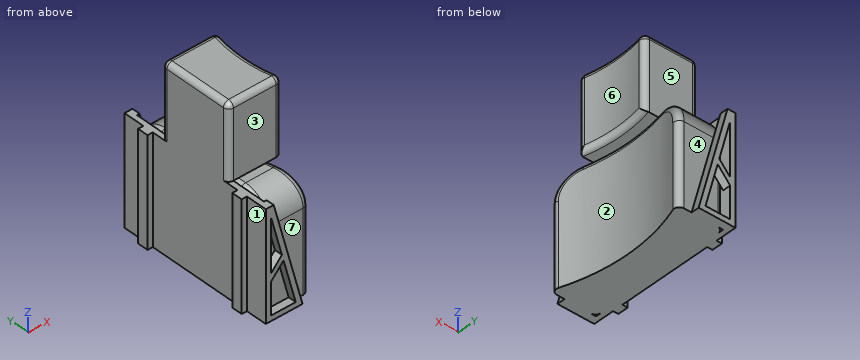
```python
from build123d import *

# Parameters (mm, degrees)
F1_DEPTH  = 15
F2_W      = 7
F2_H      = 27
F3_DEPTH  = 25
F6_DEPTH  = 20
F8_W      = 1
F8_H      = 2
F9_DEPTH  = 20.5262794416
F10_W     = 9
F10_H     = 27
F11_DEPTH = 20.5262794416
F12_R     = 35.75
F13_DEPTH = 30
F15_R     = 5
F16_R     = 1
F17_W     = 11
F17_H     = 14
F18_DEPTH = 14
F19_R     = 27.5
F20_DEPTH = 60
F22_R     = 1


with BuildPart() as f1:
    # F0 (on Front) → F1 (new body, symmetric)
    with BuildSketch(Plane.XZ):
        Polygon((0, 20.5262794416), (0, 0), (7, 0), (1.5, 20.5262794416), align=None)
    extrude(amount=F1_DEPTH, both=True)


with BuildPart() as f3:
    # F2 (on Top) → F3 (new body)
    with BuildSketch(Plane.XY):
        with Locations((4.5, 0)):
            Rectangle(F2_W, F2_H)
    extrude(amount=F3_DEPTH)


with BuildPart() as f6:
    # F4 (on Front) → F6 (new body, symmetric)
    with BuildSketch(Plane.XZ):
        Polygon((3.0705523608, 10.8011949299), (1, 18.5286015403), (1, 8.5286015403), align=None)
    extrude(amount=F6_DEPTH, both=True)


with BuildPart() as f6b:
    # F5 (on Front) → F6, piece 2 (new body, symmetric)
    with BuildSketch(Plane.XZ):
        Polygon((3.377991262, 9.6538173306), (1, 7.0437856671), (1, 1), (5.6967746272, 1), align=None)
    extrude(amount=F6_DEPTH, both=True)


with BuildPart() as f1_1:
    add(f1.part)

    # F7: cut F6b, F6, F3
    add(f6b.part, mode=Mode.SUBTRACT)
    add(f6.part, mode=Mode.SUBTRACT)
    add(f3.part, mode=Mode.SUBTRACT)

    # F8 (on face) → F9 (join, through all)
    with BuildSketch(Plane.XY.offset(20.5262794416)):
        with Locations((-0.5, -10)):
            Rectangle(F8_W, F8_H)
        with Locations((-0.5, 10)):
            Rectangle(F8_W, F8_H)
    extrude(amount=-F9_DEPTH)



with BuildPart() as f11:
    # F10 (on Top) → F11 (new body, through all)
    with BuildSketch(Plane.XY):
        with Locations((5.5, 0)):
            Rectangle(F10_W, F10_H)
    extrude(amount=F11_DEPTH)


with BuildPart() as f13:
    # F12 (on Top) → F13 (new body)
    with BuildSketch(Plane.XY):
        with Locations((43, 0)):
            Circle(F12_R)
    extrude(amount=F13_DEPTH)


with BuildPart() as f11_1:
    add(f11.part)

    # F14: cut F13
    add(f13.part, mode=Mode.SUBTRACT)

    # F15
    f15_edges = [f11_1.edges().sort_by_distance(p)[0] for p in [
        (5.448471, -13.5, 20.526279),
        (5.448471, 13.5, 20.526279),
    ]]
    fillet(f15_edges, radius=F15_R)

    # F16
    f16_edges = [f11_1.edges().sort_by_distance(p)[0] for p in [
        (9.896941, -13.5, 7.76314),
        (1, -13.5, 7.76314),
    ]]
    fillet(f16_edges, radius=F16_R)


with BuildPart() as f1_2:
    add(f1_1.part)

    add(f11_1.part)  # F18 merges F11
    # F17 (on face) → F18 (join)
    with BuildSketch(Plane.XY.offset(20.5262794416)):
        with Locations((5.5, 0)):
            Rectangle(F17_W, F17_H)
    extrude(amount=F18_DEPTH)


with BuildPart() as f20:
    # F19 (on Top) → F20 (new body)
    with BuildSketch(Plane.XY):
        with Locations((37, 0)):
            Circle(F19_R)
    extrude(amount=F20_DEPTH)


with BuildPart() as f1_3:
    add(f1_2.part)

    # F21: cut F20
    add(f20.part, mode=Mode.SUBTRACT)

    # F22
    f22_edges = [f1_3.edges().sort_by_distance(p)[0] for p in [
        (10.405828, 7, 27.526279),
        (9.5, 0, 20.526279),
        (10.405828, -7, 27.526279),
        (9.5, 0, 34.526279),
        (5.202914, 7, 34.526279),
        (5.202914, -7, 34.526279),
        (0, 0, 34.526279),
        (0, 7, 27.526279),
        (0, -7, 27.526279),
    ]]
    fillet(f22_edges, radius=F22_R)


solid = f1_3.part
```
Model file for the job. Use its own axes, mm. Face numbers are marked on the shaded views. A direction names the side the tool comes from. Give positions to 0.01 mm unless a question says otherwise; leave off trailing zeros. Loops run counter-clockwise (first coordinate to the right, second up) from the corner with the lowest first, then second, coordinate; pieces in that order, holes last. Notation, with made-up numbers: M 65,75.5 L 77,75.5 A21 ccw 77,110.5 Z; hole C 2.25,19.5 d9. An arc over 180 degrees is marked long. Use one line per item in the form item = value.
Item 1: Which spindle directions (+Z, -Z, +X, -X, +Y, -Y) get a long thin tool onto all of the face, cutting with end or side? Do the marked faces 1, 2, 3 and 4. Say none if no direction does.
Filled in:
face_1 = +Z, -Z, -X, -Y
face_2 = -Z, +X
face_3 = +Z, +X, -X, -Y
face_4 = +Z, +X, +Y
Item 2: Flat gauge pins, fed straight in: pin 1 Ø1.2 at (x, y) = (5.5, -8) entering from +Z; pin 2 Ø1.5 at (x, z) = (4.5, 23) entering from -Y; pin 3 Ø4 at (y, z) = (2.5, 25) entering from +X. Where does each tip first touch, or does it go through?
Filled in:
pin_1 = 20.53
pin_2 = -7
pin_3 = 9.87
Item 3: Drill centre lines: L1, parallel to Y at x = -0.25, z = 10.5; L2, parallel to X at y = 8.5, z = 12.5; L3, parallel to X at y = -9.5, z = 10. Where is each one in solid material? Low to high.
Filled in:
L1 = -11 to -9, 9 to 11
L2 = 0 to 8.28
L3 = -1 to 8.54
Item 4: Two-plate mould, pull along Y, no slides. Class the marked faces 5, 6 and 7: released by +Y, released by -Y, zero draft, split by the parting line, or undercut.
Filled in:
face_5 = released by +Y
face_6 = undercut
face_7 = released by -Y
Item 5: Slice it at C-C on z = 14. List the corners of the cut face in (x, y).
Filled in:
outline = M -1,-11 L 0,-11 L 0,-15 L 1,-15 L 1,-12.5 A1 ccw 2,-13.5 L 2.21,-13.5 L 2.21,-15 L 3.25,-15 L 3.25,-13.5 L 8.44,-13.5 A1 ccw 9.38,-12.16 A35.75 cw 9.38,12.16 A1 ccw 8.44,13.5 L 3.25,13.5 L 3.25,15 L 2.21,15 L 2.21,13.5 L 2,13.5 A1 ccw 1,12.5 L 1,15 L 0,15 L 0,11 L -1,11 L -1,9 L 0,9 L 0,-9 L -1,-9 Z
Item 6: Slice it at A-A on z = 22.5. List the corners of the cut face in (x, y), and give its area (3 significant figures).
Filled in:
outline = M 0,-6 A1 ccw 1,-7 L 9.14,-7 A1 ccw 10.12,-5.79 A27.5 cw 10.12,5.79 A1 ccw 9.14,7 L 1,7 A1 ccw 0,6 Z
area = 136 mm^2
Item 7: Slice it at B-B on x = 4. List the corners of the cut face in (y, z), and give its area (3 significant figures).
Filled in:
outline = M -15,0 L 15,0 L 15,1 L 13.5,1 L 13.5,7.33 L 15,7.33 L 15,11.2 L 13.5,11.2 L 13.5,15.53 A5 ccw 8.5,20.53 L 7,20.53 L 7,33.53 A1 ccw 6,34.53 L -6,34.53 A1 ccw -7,33.53 L -7,20.53 L -8.5,20.53 A5 ccw -13.5,15.53 L -13.5,11.2 L -15,11.2 L -15,7.33 L -13.5,7.33 L -13.5,1 L -15,1 Z
area = 754 mm^2
